Design review of the part built by this model. Coordinates are the model's own, in mm. Face numbers are marked on the shaded views. Round coordinates to 2 decimals unless told otherwise and drop trailing zeros. Loops run counter-clockwise (first coordinate to the right, second up) from the corner with the lowest first, then second, coordinate; pieces in that order, holes last. Notation, with made-up numbers: (88, 51.5) - (126, 51.5) arc R35 ccw to (126, 90.5) - close; hole circle Ø8 at (20.25, 0.25). An arc over 180 degrees is marked (long way). Return JSON: item names as keys, results as strings. Group by question number.
(1) Wall thickness on L1, parallel to Z at x = -2.5, y = 2.4; L2, parallel to X at y = 0.2, z = -2; L3, parallel to X at y = 1.7, z = -11: over which ranges is each line inside the solid? List them lowest first. Write a range as [from, to].
(2) The part is to be moulded in two halves that separate along X. For the marked faces 1 and 2, say which applies: pulls with the +X half, pulls with the -X half, needs draft (parallel to the pull), parting line crosses it, or undercut.
(3) Clearance check with flat-ended pins moving along their axes: pin 1 (0.5 mm diameter, centred on x = -5, y = 2, fed in from -Z); pin 2 (1.5 mm diameter, centred on x = -15.5, y = 2, fed in from -Z); pin 3 (0.7 mm diameter, centred on x = -3, y = 2, fed in from +Z). State where each tip first meets the part, or that it passes through.
(4) We need section A-A, the plane x = -5. Write out the cut boundary in (y, z), and give its area (3 significant figures).
(5) We need section B-B, the plane z = -16. Write out the cut boundary in (x, y), and give its area (3 significant figures).
(6) We need section C-C, the plane x = -16. Write out the cut boundary in (y, z).
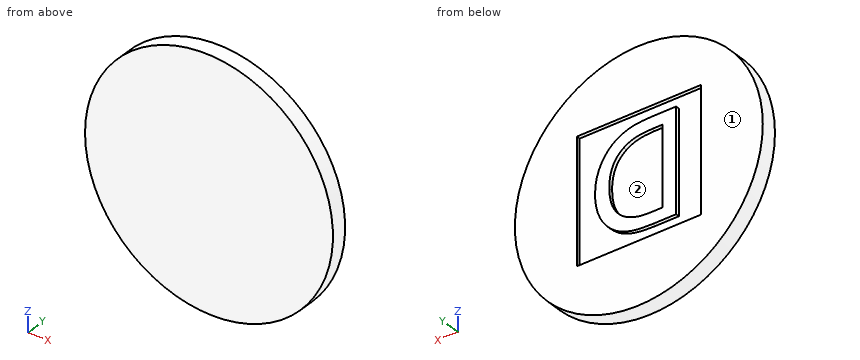
Autodesk Inventor part; units mm, degrees
ref_plane "YZ Plane" through (0, 0, 0) normal (1, 0, 0) x (0, 1, 0)
ref_plane "XZ Plane" through (0, 0, 0) normal (0, 1, 0) x (-1, 0, 0)
ref_plane "XY Plane" through (0, 0, 0) normal (0, 0, 1) x (1, 0, 0)
sketch "Sketch1" plane through (0, 0, 0) normal (0, 1, 0) x (-1, 0, 0)
  circle A0 centre (0, 0) radius 20
  dimension "d0" = 40
extrude "Extrusion1" add sketch "Sketch1" along normal blind 2.6
sketch "Sketch2" plane through (0, 2.6, 0) normal (0, 1, 0) x (1, 0, 0)
  line L0 (-10, -10) -> (-10, 10)
  line L1 (-10, 10) -> (10, 10)
  line L2 (10, 10) -> (10, -10)
  line L3 (10, -10) -> (-10, -10)
  line L4 (-10, -10) -> (10, 10) construction
  line L5 (-10, 10) -> (10, -10) construction
  point P0 (0, 0)
  dimension "d3" = 20
  dimension "d4" = 20
extrude "Extrusion2" cut sketch "Sketch2" against normal blind 0.6
sketch "Sketch3" plane through (0, 2, 0) normal (0, 1, 0) x (1, 0, 0)
  line L0 (-7.7054, 8.3364) -> (7.7781, 8.3364) construction
  line L1 (7.7781, 8.3364) -> (7.7781, -8.2636) construction
  line L2 (7.7781, -8.2636) -> (-7.7054, -8.2636) construction
  line L3 (-7.7054, -8.2636) -> (-7.7054, 8.3364) construction
  spline S0 degree 2 poles (7.0651, 0.0229) (7.0651, -2.2505) (5.2222, -5.9095) (3.6752, -6.9319) knots 0 0 0 1 2 2 2
  spline S1 degree 2 poles (3.6752, -6.9319) (2.4107, -7.7256) (-0.1856, -8.2636) (-2.2034, -8.2636) knots 0 0 0 1 2 2 2
  line L4 (-2.2034, -8.2636) -> (-6.0239, -8.2636)
  line L5 (-6.0239, -8.2636) -> (-6.0239, 8.3364)
  line L6 (-6.0239, 8.3364) -> (-2.2438, 8.3364)
  spline S2 degree 2 poles (-2.2438, 8.3364) (0.0969, 8.3364) (2.7604, 7.6368) (3.7021, 7.018) knots 0 0 0 1 2 2 2
  spline S3 degree 2 poles (3.7021, 7.018) (5.3029, 5.9553) (7.0651, 2.4443) (7.0651, 0.0229) knots 0 0 0 1 2 2 2
  spline S4 degree 2 poles (4.7648, 0.0498) (4.7648, 1.96) (3.5003, 4.6639) (2.2492, 5.4307) knots 0 0 0 1 2 2 2
  spline S5 degree 2 poles (2.2492, 5.4307) (1.3614, 5.9553) (-0.643, 6.4261) (-2.1362, 6.4261) knots 0 0 0 1 2 2 2
  line L7 (-2.1362, 6.4261) -> (-3.8177, 6.4261)
  line L8 (-3.8177, 6.4261) -> (-3.8177, -6.3534)
  line L9 (-3.8177, -6.3534) -> (-2.1362, -6.3534)
  spline S6 degree 2 poles (-2.1362, -6.3534) (-0.6699, -6.3534) (1.5497, -5.8826) (2.451, -5.2504) knots 0 0 0 1 2 2 2
  spline S7 degree 2 poles (2.451, -5.2504) (3.6079, -4.4701) (4.7648, -1.8873) (4.7648, 0.0498) knots 0 0 0 1 2 2 2
  point P0 (0, 0)
extrude "Extrusion3" add sketch "Sketch3" along normal blind 0.6
properties part number "TopMarkerPreset"
Solutions:
{
 "1": {"L1": "[-19.84, -10], [-8.34, -6.43], [6.35, 8.26], [10, 19.84]", "L2": "[-19.9, 19.9]", "L3": "[-16.7, 16.7]"},
 "2": {"face 1": "needs draft", "face 2": "undercut"},
 "3": {"pin 1": "z = -19.43", "pin 2": "z = -13.51", "pin 3": "z = 19.82"},
 "4": {"outline": "(0, -19.36) - (2.6, -19.36) - (2.6, -10) - (2, -10) - (2, -8.34) - (2.6, -8.34) - (2.6, 8.26) - (2, 8.26) - (2, 10) - (2.6, 10) - (2.6, 19.36) - (0, 19.36) - close", "area": "98.7 mm^2"},
 "5": {"outline": "(-12, 0) - (12, 0) - (12, 2.6) - (-12, 2.6) - close", "area": "62.4 mm^2"},
 "6": {"outline": "(0, -12) - (2.6, -12) - (2.6, 12) - (0, 12) - close"}
}
